from build123d import *
from build123d.topology import SkipClean

# Parameters (mm, degrees)
SKETCH_2_R                           = 20
CUT_EXTRUDE_1_DEPTH                  = 10
PATTERN_CIRCULAR_1_COUNT             = 3
CUT_EXTRUDE_START                    = -10
CUT_EXTRUDE_2_DEPTH                  = 10
PATTERN_CIRCULAR_2_COUNT             = 3
SKETCH_4_R                           = 1.5
EXTRUDE_1_DEPTH                      = 9
PATTERN_CIRCULAR_3_COUNT             = 3
SKETCH_5_W                           = 6.1
SKETCH_5_H                           = 4.309181557
CUT_EXTRUDE_3_DEPTH                  = 1.5
PATTERN_CIRCULAR_4_COUNT             = 3
CUT_EXTRUDE_4_DEPTH                  = 9
PATTERN_CIRCULAR_5_COUNT             = 3
EXTRUDE_START                        = -6.5
EXTRUDE_2_DEPTH                      = 6.5
SKETCH_9_R                           = 0.8
CUT_EXTRUDE_7_DEPTH                  = 6.4
CHAMFER_3_SIZE                       = 0.7
PATTERN_CIRCULAR_8_COUNT             = 3
CHAMFER_3_OF_PATTERN_CIRCULAR_8_SIZE = 0.7
FILLET_2_R                           = 1
FILLET_3_R                           = 1
CHAMFER_4_SIZE                       = 0.3


with BuildPart() as part:
    # 草图1 → 旋转1 (revolve)
    with BuildSketch(Plane.XY, mode=Mode.PRIVATE) as revolve_1_sk:
        Polygon((-7, 6.5), (-5, 6.5), (-5, 16.5), (0, 16.5), (0, 2.1), (-2.5, 2.1), (-2.5, 4), (-7, 4), align=None)
    revolve(revolve_1_sk.sketch.rotate(Axis((-65.742857143, 0, 0), (1, 0, 0)), 90), axis=Axis((-65.742857143, 0, 0), (1, 0, 0)))

    # 草图2 → 切除-拉伸1 (cut)
    with BuildSketch(Plane.ZY.offset(5)):
        with Locations((-25, 14.43375673)):
            Circle(SKETCH_2_R)
    cut_extrude_1 = extrude(amount=-CUT_EXTRUDE_1_DEPTH, mode=Mode.SUBTRACT)

    # 阵列(圆周)1: 切除-拉伸1 ×3 about axis
    pattern_circular_1_axis = Axis((0, 0, 0), (1, 0, 0))
    for i in range(1, PATTERN_CIRCULAR_1_COUNT):
        add(cut_extrude_1.rotate(pattern_circular_1_axis, i * 360 / PATTERN_CIRCULAR_1_COUNT), mode=Mode.SUBTRACT)

    # 草图3 → 切除-拉伸2 (cut)
    with BuildSketch(Plane.ZY.offset(5).offset(CUT_EXTRUDE_START)):
        with BuildLine():
            Line((-2.9, 8.730979327), (-2.9, 5.817215829))
            ThreePointArc((-2.9, 5.817215829), (0, 6.5), (2.9, 5.817215829))
            Line((2.9, 5.817215829), (2.9, 8.730979327))
            ThreePointArc((2.9, 8.730979327), (0, 9.2), (-2.9, 8.730979327))
        make_face()
    cut_extrude_2 = extrude(amount=CUT_EXTRUDE_2_DEPTH, mode=Mode.SUBTRACT)

    # 阵列(圆周)2: 切除-拉伸2 ×3 about axis
    pattern_circular_2_axis = Axis((0, 0, 0), (1, 0, 0))
    for i in range(1, PATTERN_CIRCULAR_2_COUNT):
        add(cut_extrude_2.rotate(pattern_circular_2_axis, i * 360 / PATTERN_CIRCULAR_2_COUNT), mode=Mode.SUBTRACT)

    # 草图4 → 凸台-拉伸1 (add)
    with BuildSketch(Plane.ZY.offset(5)):
        with BuildLine():
            Line((-5.040834524, 15.711142139), (-5.040834524, 12.511142139))
            Line((-5.040834524, 12.511142139), (-2.619572509, 12.511142139))
            ThreePointArc((-2.619572509, 12.511142139), (0, 10.7), (2.619572509, 12.511142139))
            Line((2.619572509, 12.511142139), (5.040834524, 12.511142139))
            Line((5.040834524, 12.511142139), (5.040834524, 15.711142139))
            ThreePointArc((5.040834524, 15.711142139), (0, 16.5), (-5.040834524, 15.711142139))
        make_face()
        with Locations((0, 13.5)):
            Circle(SKETCH_4_R, mode=Mode.SUBTRACT)
    extrude_1 = extrude(amount=EXTRUDE_1_DEPTH)

    # 阵列(圆周)3: 凸台-拉伸1 ×3 about axis
    pattern_circular_3_axis = Axis((0, 0, 0), (1, 0, 0))
    for i in range(1, PATTERN_CIRCULAR_3_COUNT):
        add(extrude_1.rotate(pattern_circular_3_axis, i * 360 / PATTERN_CIRCULAR_3_COUNT))

    # 草图5 → 切除-拉伸3 (cut)
    with BuildSketch(Plane.ZY.offset(14)):
        with Locations((0, 11.445409222)):
            Rectangle(SKETCH_5_W, SKETCH_5_H)
    cut_extrude_3 = extrude(amount=-CUT_EXTRUDE_3_DEPTH, mode=Mode.SUBTRACT)

    # 阵列(圆周)4: 切除-拉伸3 ×3 about axis
    pattern_circular_4_axis = Axis((0, 0, 0), (1, 0, 0))
    for i in range(1, PATTERN_CIRCULAR_4_COUNT):
        add(cut_extrude_3.rotate(pattern_circular_4_axis, i * 360 / PATTERN_CIRCULAR_4_COUNT), mode=Mode.SUBTRACT)

    # 草图6 → 切除-拉伸4 (cut)
    with BuildSketch(Plane(origin=(0, 0, 0), x_dir=(0, 0, -1), z_dir=(1, 0, 0))):
        with BuildLine():
            Line((-2.5, 16.30950643), (-2.5, 13.5))
            ThreePointArc((-2.5, 13.5), (0, 11), (2.5, 13.5))
            Line((2.5, 13.5), (2.5, 16.30950643))
            ThreePointArc((2.5, 16.30950643), (0, 16.5), (-2.5, 16.30950643))
        make_face()
    cut_extrude_4 = extrude(amount=-CUT_EXTRUDE_4_DEPTH, mode=Mode.SUBTRACT)

    # 阵列(圆周)5: 切除-拉伸4 ×3 about axis
    pattern_circular_5_axis = Axis((0, 0, 0), (1, 0, 0))
    for i in range(1, PATTERN_CIRCULAR_5_COUNT):
        add(cut_extrude_4.rotate(pattern_circular_5_axis, i * 360 / PATTERN_CIRCULAR_5_COUNT), mode=Mode.SUBTRACT)

    # 草图7 → 凸台-拉伸2 (add)
    with BuildSketch(Plane.ZY.offset(5).offset(EXTRUDE_START)):
        with BuildLine():
            Line((-5, 15.576696831), (-5, 15.724185194))
            ThreePointArc((-5, 15.724185194), (-5.448667451, 15.574402814), (-5.892857143, 15.411821265))
            ThreePointArc((-5.892857143, 15.411821265), (-4.546023726, 10.618261242), (-5, 15.576696831))
        make_face()
    extrude_2 = extrude(amount=EXTRUDE_2_DEPTH)

    # 草图9 → 切除-拉伸7 (cut)
    with SkipClean():  # the faces are left unmerged after this step: merging them gives an invalid solid
        with BuildSketch(Plane(origin=(1.5, 0, 0), x_dir=(0, 0, -1), z_dir=(1, 0, 0))):
            with Locations((5, 13.076696831)):
                Circle(SKETCH_9_R)
        cut_extrude_7 = extrude(amount=-CUT_EXTRUDE_7_DEPTH, mode=Mode.SUBTRACT)

    # 倒角3
    chamfer_3_edges = [part.edges().sort_by_distance(p)[0] for p in [
        (1.5, 13.076696831, -4.2),
    ]]
    chamfer(chamfer_3_edges, length=CHAMFER_3_SIZE)

    # 阵列(圆周)8: 凸台-拉伸2, 切除-拉伸7 ×3 about axis
    with SkipClean():  # the faces are left unmerged after this step: merging them gives an invalid solid
        pattern_circular_8_axis = Axis((0, 0, 0), (1, 0, 0))
        add([extrude_2.rotate(pattern_circular_8_axis, i * 360 / PATTERN_CIRCULAR_8_COUNT) for i in range(1, PATTERN_CIRCULAR_8_COUNT)])
        add([cut_extrude_7.rotate(pattern_circular_8_axis, i * 360 / PATTERN_CIRCULAR_8_COUNT) for i in range(1, PATTERN_CIRCULAR_8_COUNT)], mode=Mode.SUBTRACT)

    # 倒角3 of 阵列(圆周)8
    chamfer_3_of_pattern_circular_8_edges = [part.edges().sort_by_distance(p)[0] for p in [
        (1.5, -2.901041719, 13.424751653),
        (1.5, -10.175655111, -9.224751653),
    ]]
    chamfer(chamfer_3_of_pattern_circular_8_edges, length=CHAMFER_3_OF_PATTERN_CIRCULAR_8_SIZE)

    # 圆角2
    fillet_2_edges = [part.edges().sort_by_distance(p)[0] for p in [
        (-5, 12.511142139, -3.830203516),
        (-5, 10.7, 0),
        (-5, 12.511142139, 3.830203516),
    ]]
    fillet(fillet_2_edges, radius=FILLET_2_R)

    # 圆角3
    fillet_3_edges = [part.edges().sort_by_distance(p)[0] for p in [
        (-5, -9.572624616, -8.919865164),
        (-5, -5.35, -9.26647182),
        (-5, -2.938517523, -12.750068681),
        (-5, -2.938517523, 12.750068681),
        (-5, -5.35, 9.26647182),
        (-5, -9.572624616, 8.919865164),
    ]]
    fillet(fillet_3_edges, radius=FILLET_3_R)

    # 倒角4
    chamfer_4_edges = [part.edges().sort_by_distance(p)[0] for p in [
        (-7, 0, -4),
    ]]
    chamfer(chamfer_4_edges, length=CHAMFER_4_SIZE)


solid = part.part
Could you check a few things on this model? Use its own coordinates, in mm. A direction names the side the tool comes from. Give positions to 0.01 mm unless a question says otherwise; leave off trailing zeros. Write each loop counter-clockwise with the first axis right and the second up, starting at its lowest first coordinate (ties: lowest second). Pieces come first, ordered by that corner, then holes. Notation, with made-up numbers: (76.25, 45.25) -> (87.25, 45.25) arc R11 ccw to (87.25, 57.25) -> close; hole circle Ø5 at (17, 1). An arc over 180 degrees is marked (long way). Answer as a JSON object with one key per item and string values.
Q1. We'd pull the mould along Z, two halves only. Please class faces 1 (the flat face through (-12.5, -6, 10)), 2 (the flat face through (-14, -8, -13)), 3 (the flat face through (-9.44, -2.66, -14.69)), 4 (the flat face through (-12.5, 11.8, 0)): released by +Z, released by -Z, zero draft, split by the parting line, or undercut.
Taken from the geometry:
{"face 1": "undercut", "face 2": "zero draft", "face 3": "released by -Z", "face 4": "undercut"}
Q2. Suppose I cut it at B-B on x = -3.25. Count the separate pieces of the cut face and the enclosed holes in it, then the cut area to 3 significant figures.
Taken from the geometry:
{"separate pieces": "1", "enclosed holes": "7", "area": "359 mm²"}
Q3. Suppose I cut it at A-A on z = 7. Write out the boundary of the cut face in (x, y), then the cut area to 3 significant figures.
Taken from the geometry:
{"outline": "(-5, -10.13) -> (0, -10.13) -> (0, -5.97) -> (-5, -5.97) -> close; (-5, -0.69) -> (0, -0.69) -> (0, 5.72) -> (-5, 5.72) -> close", "area": "52.9 mm²"}
Q4. Will these pins go through, and if not, where does the flat tip stop? pin 1 Ø4 at (x, z) = (-1.5, -9) entering from +Y; pin 2 Ø0.9 at (x, y) = (-1.5, 7.5) entering from -Z; pin 3 Ø0.8 at (x, y) = (-2.5, 14.5) entering from +Z; pin 4 Ø2.5 at (y, z) = (0, 0) entering from +X.
Taken from the geometry:
{"pin 1": "stops at y = 14.58", "pin 2": "stops at z = -6.41", "pin 3": "stops at z = 5.01", "pin 4": "passes through"}
Q5. Which directions (+Z, -Z, +X, -X, +Y, -Y) give clear straight access to the entire face, cutting with the end or side of a thin tool? Please do faces 5 (the flat face through (-9, -8, 13)), 6 (the cylindrical face through (-5.3, -9.42, -8.68)), 7 (the flat face through (-13.26, -9.165, 9.775)), 8 (the cylindrical face through (-10.909, 14.765, 0.806)).
Taken from the geometry:
{"face 5": "+X", "face 6": "-X", "face 7": "-X, +Y", "face 8": "+X, -X"}
Q6. Please list where these lines run through material, in increasing order: L1, parallel to Y at x = -0.5, z = -0.5; L2, parallel to Y at x = -12.4, z = 0; L3, parallel to Z at x = -0.5, y = -6.5.
Taken from the geometry:
{"L1": "y = -8.87 to -2.04, 2.04 to 6.48, 9.19 to 11.05", "L2": "y = 10.7 to 12, 15 to 16.5", "L3": "z = -9.2 to -6.51, -5.46 to 5.46, 6.51 to 9.2"}
